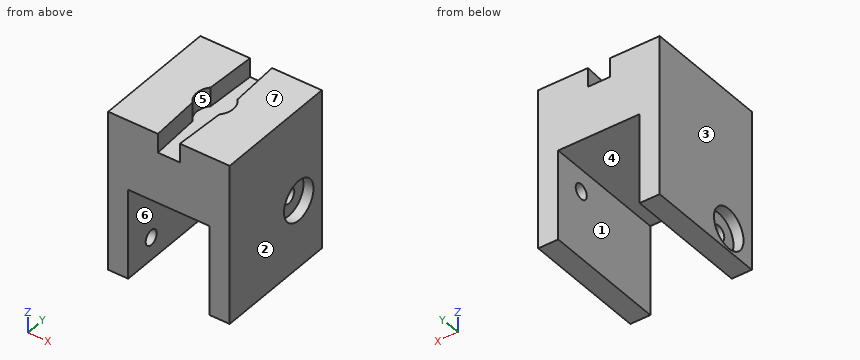
```python
from build123d import *

# Parameters (mm, degrees)
EXTRUDE_THIN1_DEPTH = 25
SKETCH2_W           = 24.3
SKETCH2_H           = 25
BOSS_EXTRUDE1_DEPTH = 10
CUT_EXTRUDE1_DEPTH  = 3.8
SKETCH4_R           = 3.65
CUT_EXTRUDE2_DEPTH  = 3.8
SKETCH5_R           = 1.5
CUT_EXTRUDE3_DEPTH  = 37.892953257
SKETCH7_R           = 1.5
CUT_EXTRUDE4_DEPTH  = 37.892953257
SKETCH8_R           = 4
CUT_EXTRUDE5_DEPTH  = 2
SKETCH9_R           = 4
CUT_EXTRUDE6_DEPTH  = 2


with BuildPart() as part:
    # Sketch1 → Extrude-Thin1 (new body)
    with BuildSketch(Plane(origin=(0, 0, 0), x_dir=(1, 0, 0), z_dir=(0, 1, 0))):
        Polygon((-8.15, 18), (-8.15, 0), (8.15, 0), (8.15, 18), (12.15, 18), (12.15, -4), (-12.15, -4), (-12.15, 18), align=None)
    extrude(amount=EXTRUDE_THIN1_DEPTH)

    # Sketch2 → Boss-Extrude1 (add)
    with BuildSketch(Plane.XY.offset(4)):
        with Locations((0, 12.5)):
            Rectangle(SKETCH2_W, SKETCH2_H)
    extrude(amount=BOSS_EXTRUDE1_DEPTH)

    # Sketch3 → Cut-Extrude1 (cut)
    with BuildSketch(Plane.XY.offset(14)):
        with BuildLine():
            Line((-2.2, 25), (-2.8, 12.5))
            Line((-2.8, 12.5), (-2.2, 0))
            ThreePointArc((-2.2, 0), (0, -2.096932942), (2.2, 0))
            Line((2.2, 0), (2.8, 12.5))
            Line((2.8, 12.5), (2.2, 25))
            ThreePointArc((2.2, 25), (0, 27.096932942), (-2.2, 25))
        make_face()
    extrude(amount=-CUT_EXTRUDE1_DEPTH, mode=Mode.SUBTRACT)

    # Sketch4 → Cut-Extrude2 (cut)
    with BuildSketch(Plane.XY.offset(14)):
        with Locations((0, 12.5)):
            Circle(SKETCH4_R)
    extrude(amount=-CUT_EXTRUDE2_DEPTH, mode=Mode.SUBTRACT)

    # Sketch5 → Cut-Extrude3 (cut, through all)
    with BuildSketch(Plane.ZY.offset(-8.15)):
        with Locations((-4.5, 18.75)):
            Circle(SKETCH5_R)
    extrude(amount=-CUT_EXTRUDE3_DEPTH, mode=Mode.SUBTRACT)

    # Sketch7 → Cut-Extrude4 (cut, through all)
    with BuildSketch(Plane(origin=(-8.15, 0, 0), x_dir=(0, 0, -1), z_dir=(1, 0, 0))):
        with Locations((13.5, 6.25)):
            Circle(SKETCH7_R)
    extrude(amount=-CUT_EXTRUDE4_DEPTH, mode=Mode.SUBTRACT)

    # Sketch8 → Cut-Extrude5 (cut)
    with BuildSketch(Plane(origin=(12.15, 0, 0), x_dir=(0, 0, -1), z_dir=(1, 0, 0))):
        with Locations((4.5, 18.75)):
            Circle(SKETCH8_R)
    extrude(amount=-CUT_EXTRUDE5_DEPTH, mode=Mode.SUBTRACT)

    # Sketch9 → Cut-Extrude6 (cut)
    with BuildSketch(Plane.ZY.offset(12.15)):
        with Locations((-13.5, 6.25)):
            Circle(SKETCH9_R)
    extrude(amount=-CUT_EXTRUDE6_DEPTH, mode=Mode.SUBTRACT)


solid = part.part
```
The model under review builds one solid part; all positions refer to its coordinate system, in mm. Face numbers are marked on the shaded views. A direction names the side the tool comes from. Round coordinates to 2 decimals unless told otherwise and drop trailing zeros. Loops run counter-clockwise (first coordinate to the right, second up) from the corner with the lowest first, then second, coordinate; pieces in that order, holes last. Notation, with made-up numbers: (25, 16.25) -> (68, 16.25) arc R23 cw to (68, 39.25) -> close; hole circle Ø1 at (-6.5, -19). An arc over 180 degrees is marked (long way). Answer in a Markdown table with one row per item.
1) Consider section C-C, the plane z = -13.5. Write out the cut boundary in (x, y), plus the area to 3 significant figures.
Taken from the geometry:
| item | result |
|---|---|
| outline | (-12.15, 0) -> (-8.15, 0) -> (-8.15, 4.75) -> (-10.15, 4.75) -> (-10.15, 2.25) -> (-12.15, 2.25) -> close; (-12.15, 10.25) -> (-10.15, 10.25) -> (-10.15, 7.75) -> (-8.15, 7.75) -> (-8.15, 25) -> (-12.15, 25) -> close; (8.15, 0) -> (12.15, 0) -> (12.15, 25) -> (8.15, 25) -> close |
| area | 178 mm² |
2) Wall thickness on line 1 along X through (y, z) = (2.75, -11); line 2 along Y through (x, z) = (-8.5, -13.5); line 3 along X through (y, z) = (7.5, -16): over which ranges is each line inside the solid? List them lowest first.
Taken from the geometry:
| item | result |
|---|---|
| line 1 | x = -12.15 to -8.15, 8.15 to 12.15 |
| line 2 | y = 0 to 4.75, 7.75 to 25 |
| line 3 | x = -10.15 to -8.15, 8.15 to 12.15 |
3) Consider section D-D, the plane x = 1. Write out the cut boundary in (y, z), plus the area to 3 significant figures.
Taken from the geometry:
| item | result |
|---|---|
| outline | (0, 0) -> (25, 0) -> (25, 10.2) -> (0, 10.2) -> close |
| area | 255 mm² |
4) Draft analysis for pull direction X (two halves, no side actions). For the marked faces 1, 2, 3 and 4, state which applies: pulls with the +X half, pulls with the -X half, needs draft (parallel to the pull), parting line crosses it, or undercut.
Taken from the geometry:
| item | result |
|---|---|
| face 1 | undercut |
| face 2 | pulls with the +X half |
| face 3 | pulls with the -X half |
| face 4 | undercut |
5) Tool access review of the marked faces 5, 6 and 7: name each direction out of +Z, -Z, +X, -X, +Y, -Y from which nothing blocks a thin tool from reaching the whole face with its end or side.
Taken from the geometry:
| item | result |
|---|---|
| face 5 | +Z |
| face 6 | -Z, +Y, -Y |
| face 7 | +Z, +X, -X, +Y, -Y |
6) For pin 1 Ø2.5 at (y, z) = (7.5, -15) entering from -X; pin 2 Ø13 at (x, y) = (-0.5, 15) entering from -Z; pin 3 Ø4 at (y, z) = (20, -3) entering from +X, all flat-tipped, find the tip position at first contact; note any pin that passes through.
Taken from the geometry:
| item | result |
|---|---|
| pin 1 | stops at x = -10.15 |
| pin 2 | stops at z = 0 |
| pin 3 | stops at x = 10.15 |
7) Consider section A-A, the plane z = -9. Write out the cut boundary in (x, y), plus the area to 3 significant figures.
Taken from the geometry:
| item | result |
|---|---|
| outline | (-12.15, 0) -> (-8.15, 0) -> (-8.15, 25) -> (-12.15, 25) -> close; (8.15, 0) -> (12.15, 0) -> (12.15, 25) -> (8.15, 25) -> close |
| area | 200 mm² |
8) Consider section B-B, the plane y = 18.75. Write out the cut boundary in (x, z), plus the area to 3 significant figures.
Taken from the geometry:
| item | result |
|---|---|
| outline | (-12.15, -18) -> (-8.15, -18) -> (-8.15, 0) -> (8.15, 0) -> (8.15, -3) -> (10.15, -3) -> (10.15, -0.5) -> (12.15, -0.5) -> (12.15, 14) -> (2.5, 14) -> (2.5, 10.2) -> (-2.5, 10.2) -> (-2.5, 14) -> (-12.15, 14) -> close; (8.15, -18) -> (12.15, -18) -> (12.15, -8.5) -> (10.15, -8.5) -> (10.15, -6) -> (8.15, -6) -> close |
| area | 443 mm² |
